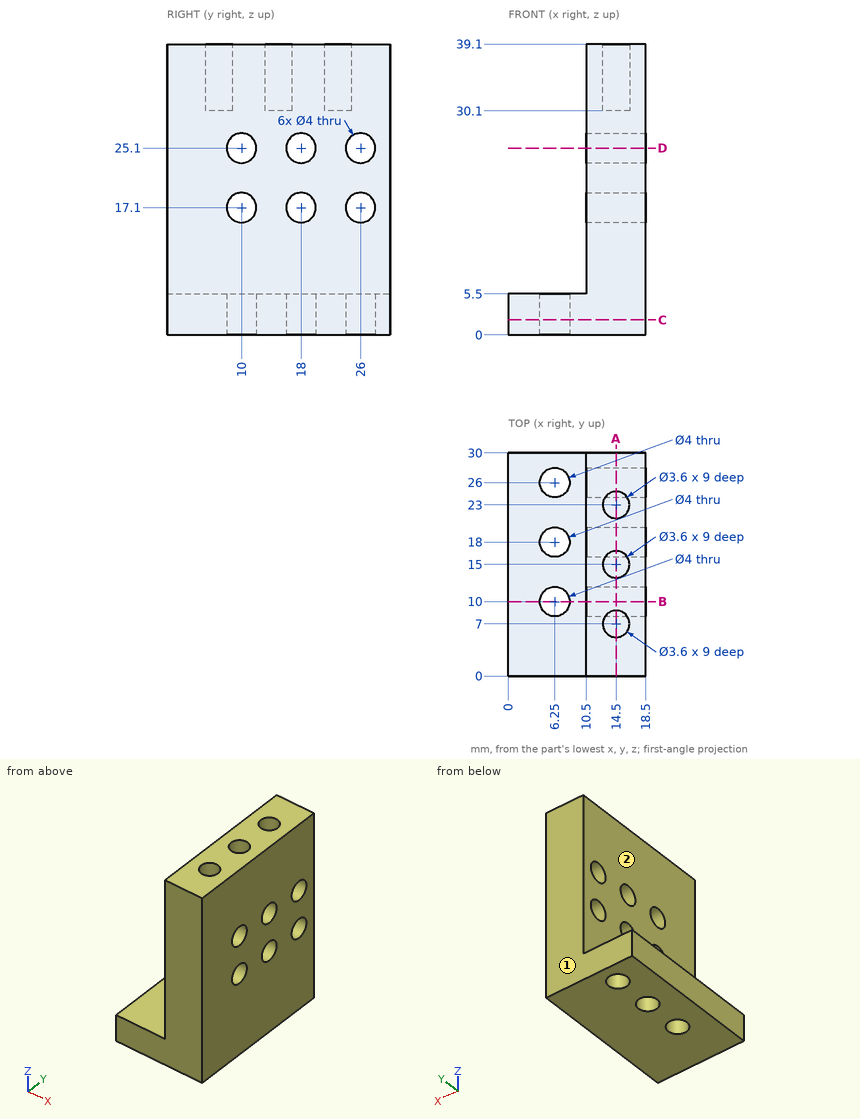
Geometry check sheet. Reference: drawing and pictorial views, mm from the part's lowest x, y, z. A direction names the side the tool comes from. Coordinates: 2 decimals unless noted, no trailing zeros. Write each loop counter-clockwise with the first axis right and the second up, starting at its lowest first coordinate (ties: lowest second). Pieces come first, ordered by that corner, then holes. Notation, with made-up numbers: (-24.5, 81.5) - (22.5, 81.5) arc R22 cw to (22.5, 92.5) - close; hole circle Ø11 at (-30, -15). An arc over 180 degrees is marked (long way). One line per question, with ' | ' between items. Start each with the question number.
1. Section check C-C (z = 2). Enter the section's corners in (x, y), plus the area to 3 significant figures.
2. Section check D-D (z = 25.1). Enter the section's corners in (x, y).
3. Section check B-B (y = 10). Enter the section's corners in (x, z).
4. Access from +Z, -Z, +X, -X, +Y, -Y to the whole of each face (thin tool, end or side, straight path). Record for the marked faces 1 and 2.
5. Section check A-A (x = 14.5). Enter the section's corners in (y, z).
6. Material ranges on line 1 along Y through (x, z) = (15.75, 17.1); line 2 along Y through (x, z) = (14.5, 36.5); line 3 along Z through (x, y) = (13.5, 17), recorded low to high.
7. Gauge pin test, flat ends, axial feed: P1, Ø3, axis at x = 2.5, y = 10, coming from the +Z side; P2, Ø5, axis at y = 26, z = 17.1, coming from the -X side; P3, Ø3, axis at y = 18, z = 25.1, coming from the -X side; P4, Ø3, axis at x = 14.5, y = 7, coming from the +Z side. Record the tip position at first contact, or that the pin passes through.
Computed values:
1) outline: (0, 0) - (18.5, 0) - (18.5, 30) - (0, 30) - close; hole circle Ø4 at (6.25, 10); hole circle Ø4 at (6.25, 18); hole circle Ø4 at (6.25, 26) | area: 517 mm²
2) outline: (10.5, 0) - (18.5, 0) - (18.5, 8) - (10.5, 8) - close; (10.5, 12) - (18.5, 12) - (18.5, 16) - (10.5, 16) - close; (10.5, 20) - (18.5, 20) - (18.5, 24) - (10.5, 24) - close; (10.5, 28) - (18.5, 28) - (18.5, 30) - (10.5, 30) - close
3) outline: (0, 0) - (4.25, 0) - (4.25, 5.5) - (0, 5.5) - close; (8.25, 0) - (18.5, 0) - (18.5, 15.1) - (10.5, 15.1) - (10.5, 5.5) - (8.25, 5.5) - close; (10.5, 19.1) - (18.5, 19.1) - (18.5, 23.1) - (10.5, 23.1) - close; (10.5, 27.1) - (18.5, 27.1) - (18.5, 39.1) - (10.5, 39.1) - close
4) face 1: +Z, -Z, +X, -X, +Y | face 2: +Z, -X, +Y, -Y
5) outline: (0, 0) - (30, 0) - (30, 39.1) - (24.8, 39.1) - (24.8, 30.1) - (21.2, 30.1) - (21.2, 39.1) - (16.8, 39.1) - (16.8, 30.1) - (13.2, 30.1) - (13.2, 39.1) - (8.8, 39.1) - (8.8, 30.1) - (5.2, 30.1) - (5.2, 39.1) - (0, 39.1) - close; hole circle Ø4 at (10, 17.1); hole circle Ø4 at (10, 25.1); hole circle Ø4 at (18, 17.1); hole circle Ø4 at (18, 25.1); hole circle Ø4 at (26, 17.1); hole circle Ø4 at (26, 25.1)
6) line 1: 0 to 8, 12 to 16, 20 to 24, 28 to 30 | line 2: 0 to 5.2, 8.8 to 13.2, 16.8 to 21.2, 24.8 to 30 | line 3: 0 to 15.37, 18.83 to 23.37, 26.83 to 39.1
7) P1: z = 5.5 | P2: x = 10.5 | P3: through | P4: z = 30.1
